from build123d import *

# Parameters (mm, degrees)
BOSS_EXTRUDE1_START = 2
SKETCH2_R           = 24.705
BOSS_EXTRUDE1_DEPTH = 2
FILLET1_R           = 10
FILLET2_R           = 10


# Read off the part's stored shape, not the designer's step: Shell2
with BuildPart() as part:
    # Sketch1 → Revolve1 (revolve)
    with BuildSketch(Plane.XY):
        with BuildLine():
            Line((-173.75, 0), (0, 0))
            Line((0, 0), (0, 15))
            Line((0, 15), (-13.19, 15))
            Line((-13.19, 15), (-50.28, 22.75))
            Line((-50.28, 22.75), (-77.37, 34.705))
            ThreePointArc((-77.37, 34.705), (-120.56, 30.423853835), (-163.75, 34.705))
            ThreePointArc((-163.75, 34.705), (-170.821067812, 31.776067812), (-173.75, 24.705))
            Line((-173.75, 24.705), (-173.75, 0))
        make_face()
    revolve(axis=Axis((0, 0, 0), (-1, 0, 0)))

    # Shell2 outline → Shell2 (revolve, cut)
    with BuildSketch(Plane.YX):
        with BuildLine():
            Line((24.705, -173.75), (24.705, -171.75))
            ThreePointArc((24.705, -171.75), (30.295405132, -169.472531822), (32.702817817, -163.936842615))
            ThreePointArc((32.702817817, -163.936842615), (28.423955347, -120.772299747), (32.620253078, -77.599652035))
            Line((32.620253078, -77.599652035), (20.835311789, -50.895004646))
            Line((20.835311789, -50.895004646), (13, -13.396718937))
            Line((13, -13.396718937), (13, 0))
            Line((13, 0), (0, 0))
            Line((0, 0), (0, -173.75))
            Line((0, -173.75), (24.705, -173.75))
        make_face()
    revolve(axis=Axis((0, 0, 0), (1, 0, 0)), mode=Mode.SUBTRACT)

    # Sketch2 → Boss-Extrude1 (add)
    with BuildSketch(Plane(origin=(-173.75, 0, 0), x_dir=(0, 0, -1), z_dir=(1, 0, 0)).offset(BOSS_EXTRUDE1_START)):
        Circle(SKETCH2_R)
    extrude(amount=-BOSS_EXTRUDE1_DEPTH)

    # Fillet1
    fillet1_edges = [part.edges().sort_by_distance(p)[0] for p in [
        (-77.37, -34.705, 0),
        (-50.28, -22.75, 0),
        (-13.19, -15, 0),
    ]]
    fillet(fillet1_edges, radius=FILLET1_R)

    # Fillet2
    fillet2_edges = [part.edges().sort_by_distance(p)[0] for p in [
        (-13.396718937, -13, 0),
    ]]
    fillet(fillet2_edges, radius=FILLET2_R)


solid = part.part
Could you check a few things on this model? Use its own coordinates, in mm. A direction names the side the tool comes from. Coordinates: 2 decimals unless noted, no trailing zeros. Loops run counter-clockwise (first coordinate to the right, second up) from the corner with the lowest first, then second, coordinate; pieces in that order, holes last. Notation, with made-up numbers: (63, 40) -> (119, 40) arc R22 ccw to (119, 56) -> close; hole circle Ø11 at (66.5, 18.25). An arc over 180 degrees is marked (long way). Answer in a Markdown table with one row per item.
(1) Thinking about a two-plate mould opening in Z: for faces 1 (the face through (-173.75, 0, 0)), 2 (the face through (-55.16, 21.67, 6.82)), 3 (the face through (-6.163, -14.985, -0.66)), which applies, released by +Z, released by -Z, zero draft, split by the parting line, or undercut?
Results found:
| item | result |
|---|---|
| face 1 | zero draft |
| face 2 | undercut |
| face 3 | split by the parting line |
(2) If I drill on probe 1 along Y at (x, z) = (-7, 0); probe 2 along Z at (x, y) = (-28, 9.5), over which ranges is the centre line in solid material (lowest first)?
Results found:
| item | result |
|---|---|
| probe 1 | y = -15 to -13, 13 to 15 |
| probe 2 | z = -15.4 to -12.94, 12.94 to 15.4 |
(3) For faces 4 (the face through (0, 0.1, -13.4)), 5 (the face through (-171.75, 0, 0)), 6 (the face through (-6.1, -2.82, -12.69)), which set-ups out of +Z, -Z, +X, -X, +Y, -Y let a thin tool reach every point of the face, with its end or its side?
Results found:
| item | result |
|---|---|
| face 4 | +Z, -Z, +X, +Y, -Y |
| face 5 | none |
| face 6 | +X |
(4) Imagine slicing it at A-A (x = -58). List the corners of the cut face in (y, z) for me.
Results found:
| item | result |
|---|---|
| outline | circle Ø52.31 at (0, 0); hole circle Ø47.94 at (0, 0) |
(5) Imagine slicing it at B-B (x = -96). List the corners of the cut face in (y, z) for me, plus the area to 3 significant figures.
Results found:
| item | result |
|---|---|
| outline | circle Ø63.6 at (0, 0); hole circle Ø59.57 at (0, 0) |
| area | 389 mm^2 |
(6) Will these pins go through, and if not, where does the flat tip stop? pin 1 Ø1 at (x, z) = (-72.5, -22) entering from +Y; pin 2 Ø1 at (x, y) = (-86.5, -26) entering from +Z; pin 3 Ø10 at (x, y) = (-75.5, 13) entering from +Z.
Results found:
| item | result |
|---|---|
| pin 1 | stops at y = 24.54 |
| pin 2 | stops at z = 21.08 |
| pin 3 | stops at z = 33.19 |
